Study the drawing (mm; zero at the part's minimum x, y, z) and answer. Round coordinates to 2 decimals unless told otherwise and drop trailing zeros. Write each loop counter-clockwise with the first axis right and the second up, starting at its lowest first coordinate (ties: lowest second). Pieces come first, ordered by that corner, then holes. Notation, with made-up numbers: M 7,23.5 L 35,23.5 A13 cw 35,38.5 Z; hole C 38,75 d2. An arc over 180 degrees is marked long. Write each question's results on one line, items separated by ' | '.
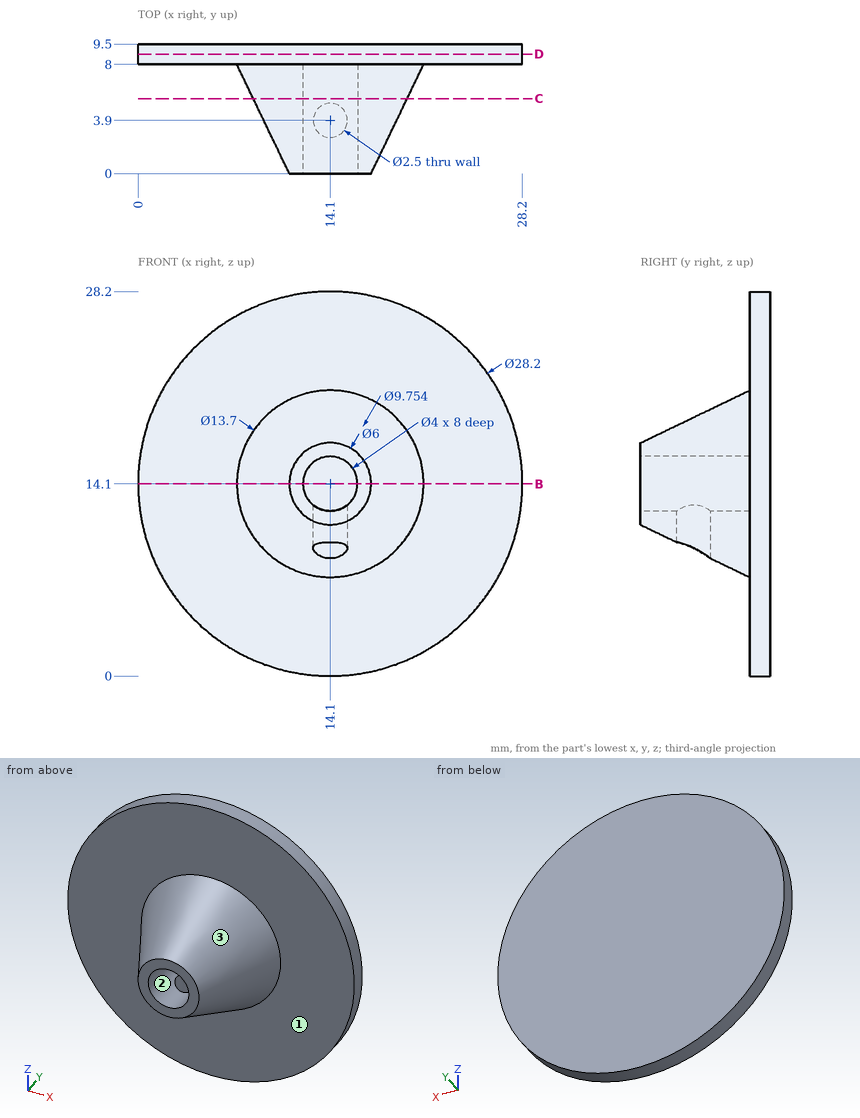
1) Section C-C (y = 5.5) is taken. Determine the outline of the cut face in (x, z), then the cut area to 3 significant figures.
Return value:
outline: C 14.1,14.1 d11.29; hole C 14.1,14.1 d4 | area: 87.6 mm²
2) The mould has two halves that part along Z. Classify the marked faces 1, 2 and 3: +Z half, -Z half, draft (parallel to the pull), parting line (faces both ways), or undercut.
Return value:
face 1: draft | face 2: undercut | face 3: parting line
3) Section B-B (z = 14.1) is taken. Determine the outline of the cut face in (x, y).
Return value:
outline: M 0,8 L 7.25,8 L 11.1,0 L 12.1,0 L 12.1,8 L 16.1,8 L 16.1,0 L 17.1,0 L 20.95,8 L 28.2,8 L 28.2,9.5 L 0,9.5 Z
4) Find the intervals of material crossed by line 1 (Y direction, x = 14.1, z = 11.3); line 2 (Z direction, x = 14.1, y = 5.5); line 3 (X direction, y = 7.5, z = 15), in increasing order.
Return value:
line 1: 0 to 2.65, 5.15 to 9.5 | line 2: 8.45 to 12.1, 16.1 to 19.75 | line 3: 7.55 to 12.31, 15.89 to 20.65
5) Each of these flat-tipped pins is pushed along its axis until it touches: pin 1 (2 mm diameter, centred on y = 7.5, z = 7, fed in from -X); pin 2 (1.2 mm diameter, centred on x = 13.5, z = 15, fed in from -Y); pin 3 (2 mm diameter, centred on x = 14.1, y = 3.9, fed in from -Z). Where does it stop, or does it pass through?
Return value:
pin 1: x = 1.45 | pin 2: y = 8 | pin 3: z = 15.83
6) Section D-D (y = 8.75) is taken. Determine the outline of the cut face in (x, z).
Return value:
outline: C 14.1,14.1 d28.2
